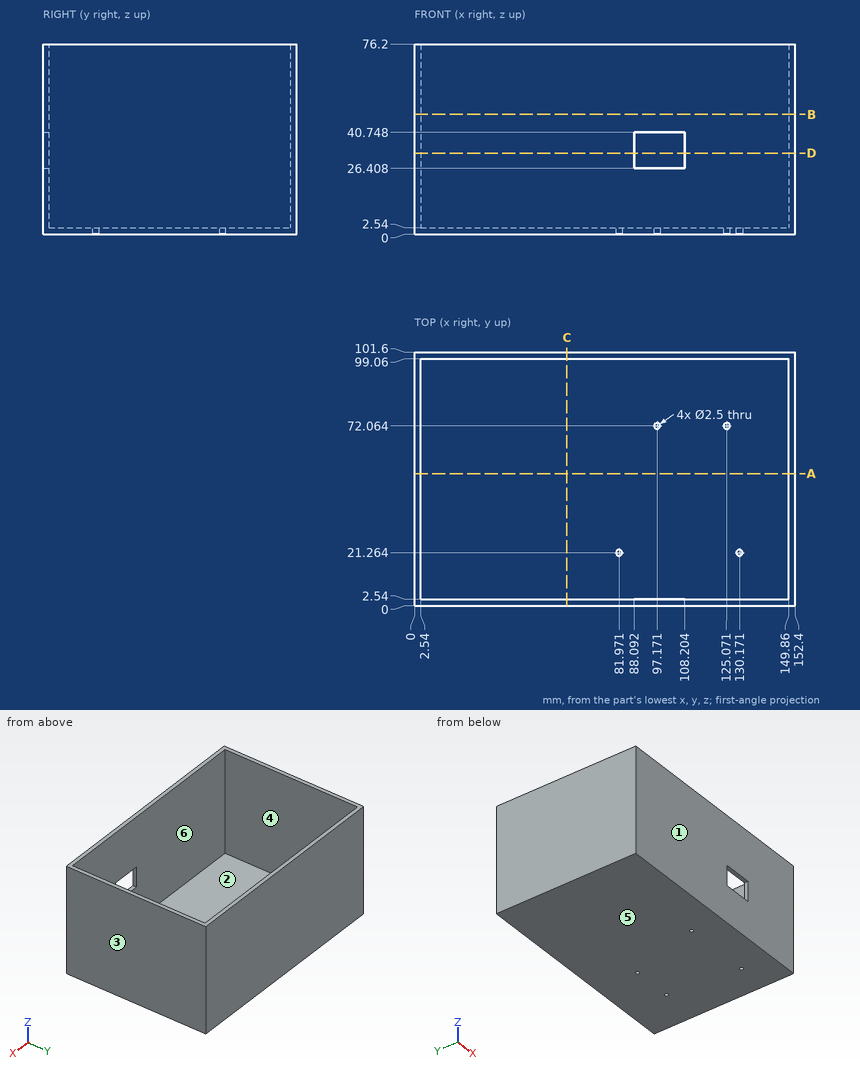
Here's the drawing with two shaded views (mm, measured from the low corner). I have some questions. A direction names the side the tool comes from. Coordinates: 2 decimals unless noted, no trailing zeros. Loops run counter-clockwise (first coordinate to the right, second up) from the corner with the lowest first, then second, coordinate; pieces in that order, holes last. Notation, with made-up numbers: M -9,82.5 L 15,82.5 A16 cw 15,95.5 Z; hole C 82,76.5 d10. An arc over 180 degrees is marked long. Return JSON: item names as keys, results as strings. Group by question number.
Item 1: Imagine slicing it at B-B (z = 48). Please give me the cut outline in (x, y).
Item 2: Imagine slicing it at A-A (y = 53). Please give me the cut outline in (x, z).
Item 3: Thinking about a two-plate mould opening in X: for the marked faces 1, 2, 3 and 4, which applies, released by +X, released by -X, zero draft, split by the parting line, or undercut?
Item 4: On a 3-axis mill with a long thin cutter (end or side, diameter ignored), from which of +Z, -Z, +X, -X, +Y, -Y can I reach the whole of each face in a straight line? I mean the marked faces 5 and 6. Say none if no direction works.
Item 5: I'm going to push a flat-ended pin straight in: pin 1 Ø2 at (x, y) = (130.17, 21.26) entering from +Z. Where does the tip first touch, or does it pass through?
Item 6: Imagine slicing it at D-D (z = 32.5). Please give me the cut outline in (x, y).
Item 7: If I drill on L1, parallel to Y at x = 114.5, z = 45; L2, parallel to X at y = 50, z = 43; L3, parallel to Z at x = 89, y = 54, over which ranges is the centre line in solid material (lowest first)? Write a range as from..to.
Item 8: Imagine slicing it at C-C (x = 61). Please give me the cut outline in (y, z).
Verdict:
{
 "1": {"outline": "M 0,0 L 152.4,0 L 152.4,101.6 L 0,101.6 Z; hole M 2.54,2.54 L 149.86,2.54 L 149.86,99.06 L 2.54,99.06 Z"},
 "2": {"outline": "M 0,0 L 152.4,0 L 152.4,76.2 L 149.86,76.2 L 149.86,2.54 L 2.54,2.54 L 2.54,76.2 L 0,76.2 Z"},
 "3": {"face 1": "zero draft", "face 2": "undercut", "face 3": "released by +X", "face 4": "undercut"},
 "4": {"face 5": "-Z, +X, -X, +Y, -Y", "face 6": "+Z"},
 "5": {"pin 1": "passes through"},
 "6": {"outline": "M 0,0 L 88.09,0 L 88.09,2.54 L 2.54,2.54 L 2.54,99.06 L 149.86,99.06 L 149.86,2.54 L 108.2,2.54 L 108.2,0 L 152.4,0 L 152.4,101.6 L 0,101.6 Z"},
 "7": {"L1": "y = 0..2.54, 99.06..101.6", "L2": "x = 0..2.54, 149.86..152.4", "L3": "z = 0..2.54"},
 "8": {"outline": "M 0,0 L 101.6,0 L 101.6,76.2 L 99.06,76.2 L 99.06,2.54 L 2.54,2.54 L 2.54,76.2 L 0,76.2 Z"}
}
